Could you check a few things on this model? Use its own coordinates, in mm. A direction names the side the tool comes from. Give positions to 0.01 mm unless a question says otherwise; leave off trailing zeros. Loops run counter-clockwise (first coordinate to the right, second up) from the corner with the lowest first, then second, coordinate; pieces in that order, holes last.
1. For faces 1 (the flat face through (9, 6, -3)), 2 (the flat face through (6, -1, 0)), 3 (the flat face through (-3, 5, -1)), 4 (the flat face through (12.25, 5, -5)), 5 (the flat face through (6, 0, 3)), which set-ups out of +Z, -Z, +X, -X, +Y, -Y let a thin tool reach every point of the face, with its end or its side?
2. I need wall thicknesses on line 1 along Y through (x, z) = (7.5, -6.65); line 2 along X through (y, z) = (4.5, -4.8); line 3 along Y through (x, z) = (7.5, -2.55). Which ranges of each line are inside material? Lowest first, please.
3. Imagine slicing it at B-B (x = 7.5). List the corners of the cut face in (y, z) for me, plus the area to 3 significant figures.
4. For P1, Ø1, axis at x = 9, y = 7, coming from the +Z side, with a flat end and sliding along its axis, tell me the tip position at first contact or that it passes through.
5. Thinking about a two-plate mould opening in Z: for faces 6 (the flat face through (12.25, 10, 3)), 7 (the flat face through (-1, 5, 6.5)), 8 (the flat face through (6, 11, 0)), which applies, +Z half, -Z half, draft (parallel to the pull), parting line (faces both ways), or undercut?
6. Imagine slicing it at C-C (z = 3.25). List the corners of the cut face in (x, y) for me.
7. Imagine slicing it at A-A (y = 4.5). List the corners of the cut face in (x, z) for me, plus the area to 3 significant figures.
8. Imagine slicing it at D-D (y = -0.75). List the corners of the cut face in (x, z) for me.
```python
from build123d import *

# Parameters (mm, degrees)
PAD_DEPTH    = 6.5
SKETCH001_W  = 15
SKETCH001_H  = 2
PAD001_DEPTH = 3
SKETCH002_W  = 15.25
SKETCH002_H  = 15
SKETCH002_R  = 1.75
PAD002_DEPTH = 6
SKETCH003_R  = 3
POCKET_DEPTH = 5


with BuildPart() as part:
    # Sketch → Pad (new body)
    with BuildSketch(Plane.XY):
        Polygon((0, 9), (12.25, 9), (12.25, 12), (-3, 12), (-3, -3), (12.25, -3), (12.25, 0), (0, 0), align=None)
    extrude(amount=PAD_DEPTH)

    # Sketch001 (on Face5 of Pad) → Pad001 (join)
    with BuildSketch(Plane(origin=(-3, 0, 0), x_dir=(0, -1, 0), z_dir=(-1, 0, 0))):
        with Locations((-4.5, -1)):
            Rectangle(SKETCH001_W, SKETCH001_H)
    extrude(amount=-PAD001_DEPTH)

    # Sketch002 (on Face11 of Pad001) → Pad002 (join)
    with BuildSketch(Plane(origin=(0, 0, -2), x_dir=(1, 0, 0), z_dir=(0, 0, -1))):
        with Locations((4.625, -4.5)):
            Rectangle(SKETCH002_W, SKETCH002_H)
        with Locations((7.5, -4.5)):
            Circle(SKETCH002_R, mode=Mode.SUBTRACT)
    extrude(amount=PAD002_DEPTH)

    # Sketch003 (on Face22 of Pad002) → Pocket (cut)
    with BuildSketch(Plane(origin=(0, 0, -8), x_dir=(1, 0, 0), z_dir=(0, 0, -1))):
        with Locations((7.5, -4.5)):
            Circle(SKETCH003_R)
    extrude(amount=-POCKET_DEPTH, mode=Mode.SUBTRACT)


solid = part.part
```
Derived:
1. face 1: -Z
1. face 2: +X, +Y, -Y
1. face 3: +Z, -Z, -X, +Y, -Y
1. face 4: +Z, -Z, +X, +Y, -Y
1. face 5: +Z, +X
2. line 1: y = -3 to 1.5, 7.5 to 12
2. line 2: x = -3 to 4.5, 10.5 to 12.25
2. line 3: y = -3 to 2.75, 6.25 to 12
3. outline: (-3, -8) - (1.5, -8) - (1.5, -3) - (2.75, -3) - (2.75, -2) - (-3, -2) - close; (-3, 0) - (0, 0) - (0, 6.5) - (-3, 6.5) - close; (6.25, -3) - (7.5, -3) - (7.5, -8) - (12, -8) - (12, -2) - (6.25, -2) - close; (9, 0) - (12, 0) - (12, 6.5) - (9, 6.5) - close
3. area: 95.5 mm2
4. P1: stops at z = -2
5. face 6: draft
5. face 7: +Z half
5. face 8: undercut
6. outline: (-3, -3) - (12.25, -3) - (12.25, 0) - (0, 0) - (0, 9) - (12.25, 9) - (12.25, 12) - (-3, 12) - close
7. outline: (-3, -8) - (4.5, -8) - (4.5, -3) - (5.75, -3) - (5.75, -2) - (0, -2) - (0, 6.5) - (-3, 6.5) - close; (9.25, -3) - (10.5, -3) - (10.5, -8) - (12.25, -8) - (12.25, -2) - (9.25, -2) - close
7. area: 83.5 mm2
8. outline: (-3, -8) - (12.25, -8) - (12.25, -2) - (0, -2) - (0, 0) - (12.25, 0) - (12.25, 6.5) - (-3, 6.5) - close
